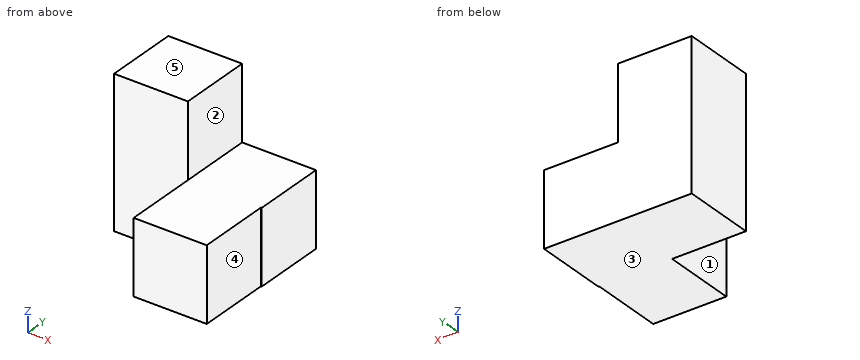
```python
from build123d import *

# Parameters (mm, degrees)
F0_W     = 19.05
F0_H     = 19.05
F1_DEPTH = 38.1
F2_W     = 19.05
F2_H     = 19.05
F3_DEPTH = 19.05
F4_W     = 18.848901
F4_H     = 19.05
F5_DEPTH = 19.05


with BuildPart() as f1:
    # F0 (on Top) → F1 (new body)
    with BuildSketch(Plane.XY):
        with Locations((-28.373901, -13.033835)):
            Rectangle(F0_W, F0_H)
    extrude(amount=F1_DEPTH)

    # F2 (on face) → F3 (join)
    with BuildSketch(Plane.YZ.offset(-18.848901)):
        with Locations((-13.033835, 9.525)):
            Rectangle(F2_W, F2_H)
    extrude(amount=F3_DEPTH)

    # F4 (on face) → F5 (join)
    with BuildSketch(Plane.XZ.offset(22.558835)):
        with Locations((-9.42445, 9.525)):
            Rectangle(F4_W, F4_H)
    extrude(amount=F5_DEPTH)


solid = f1.part
```
Part model, mm, in its own coordinate system. Face numbers are marked on the shaded views. A direction names the side the tool comes from. Round coordinates to 2 decimals unless told otherwise and drop trailing zeros. Write each loop counter-clockwise with the first axis right and the second up, starting at its lowest first coordinate (ties: lowest second). Pieces come first, ordered by that corner, then holes. Notation, with made-up numbers: M -18.75,65 L -2.75,65 A31 cw -2.75,89 Z; hole C 25.25,65.25 d5. An arc over 180 degrees is marked long. Answer as CSV lines item,"result". Start each with the question number.
1) Band-saw the part on C-C (x = -30). List the corners of the cut face in (y, z), then the cut area to 3 significant figures.
2) Band-saw the part on D-D (y = -35). List the corners of the cut face in (x, z).
3) Band-saw the part on B-B (y = -12). List the corners of the cut face in (x, z), then the cut area to 3 significant figures.
4) Drop flat-ended pins along their axis: pin 1 (5 mm diameter, centred on y = -20.5, z = 24, fed in from +X); pin 2 (9.5 mm diameter, centred on x = -27, z = 17.5, fed in from -Y); pin 3 (1 mm diameter, centred on y = -31.5, z = 15.5, fed in from -X). Give the stop position or say it passes through.
5) Drill centre lines: L1, parallel to X at y = -17.5, z = 33.5; L2, parallel to X at y = -32, z = 14; L3, parallel to Y at x = -22, z = 23. Where is each one in solid material? Low to high.
6) Which spindle directions (+Z, -Z, +X, -X, +Y, -Y) get a long thin tool onto all of the face, cutting with end or side? Do the marked faces 1, 2, 3, 4 and 5. Say none if no direction does.
7) Band-saw the part on A-A (z = 13). List the corners of the cut face in (x, y).
Worked out:
1,outline,"M -22.56,0 L -3.51,0 L -3.51,38.1 L -22.56,38.1 Z"
1,area,"726 mm²"
2,outline,"M -18.85,0 L 0,0 L 0,19.05 L -18.85,19.05 Z"
3,outline,"M -37.9,0 L 0.2,0 L 0.2,19.05 L -18.85,19.05 L -18.85,38.1 L -37.9,38.1 Z"
3,area,"1,090 mm²"
4,pin 1,"x = -18.85"
4,pin 2,"y = -22.56"
4,pin 3,"x = -18.85"
5,L1,"-37.9 to -18.85"
5,L2,"-18.85 to 0"
5,L3,"-22.56 to -3.51"
6,face 1,"+Z, -Z, -X, -Y"
6,face 2,"+Z, +X, +Y, -Y"
6,face 3,"-Z, +X, -X, +Y, -Y"
6,face 4,"+Z, -Z, +X, -Y"
6,face 5,"+Z, +X, -X, +Y, -Y"
7,outline,"M -37.9,-22.56 L -18.85,-22.56 L -18.85,-41.61 L 0,-41.61 L 0,-22.56 L 0.2,-22.56 L 0.2,-3.51 L -37.9,-3.51 Z"
